```python
from build123d import *

# Parameters (mm, degrees)
RESSALTO_EXTRUS_O1_DEPTH = 70
RESSALTO_EXTRUS_O2_REACH = 92.865
CORTE_EXTRUS_O1_DEPTH    = 70


with BuildPart() as part:
    # Esboço1 → Ressalto-extrusão1 (new body)
    with BuildSketch(Plane.XY):
        Polygon((-46.166666667, -15.652777778), (33.833333333, 19.347222222), (33.833333333, -15.652777778), align=None)
    extrude(amount=RESSALTO_EXTRUS_O1_DEPTH)

    # Ressalto-extrusão2: up to this plane
    ressalto_extrus_o2_end = Plane(origin=(-46.166666667, -15.652777778, 70), z_dir=(0.4008188340197078, -0.9161573349021892, 0))
    # Esboço3 → Ressalto-extrusão2 (add, up to the surface)
    with BuildSketch(Plane.XZ.offset(15.652777778), mode=Mode.PRIVATE) as ressalto_extrus_o2_sk1:
        with BuildLine():
            Line((-10.666666667, 70), (-1.666666667, 70))
            Line((-1.666666667, 70), (-1.666666667, 75.846688069))
            ThreePointArc((-1.666666667, 75.846688069), (-6.166666667, 85.815315035), (-10.666666667, 75.846688069))
            Line((-10.666666667, 75.846688069), (-10.666666667, 70))
        make_face()
    ressalto_extrus_o2_tool1 = split(extrude(ressalto_extrus_o2_sk1.sketch, amount=-RESSALTO_EXTRUS_O2_REACH, mode=Mode.PRIVATE), bisect_by=ressalto_extrus_o2_end, keep=Keep.BOTH, mode=Mode.PRIVATE)
    add(ressalto_extrus_o2_tool1.solids().sort_by_distance((-6.166667, -15.652778, 77.842662))[0])

    # Esboço2 → Corte-extrusão1 (cut)
    with BuildSketch(Plane.XZ.offset(15.652777778)):
        with BuildLine():
            Line((-11.166666667, 0), (-1.166666667, 0))
            Line((-1.166666667, 0), (-1.166666667, 5.846688069))
            ThreePointArc((-1.166666667, 5.846688069), (-6.166666667, 16.5), (-11.166666667, 5.846688069))
            Line((-11.166666667, 5.846688069), (-11.166666667, 0))
        make_face()
    extrude(amount=-CORTE_EXTRUS_O1_DEPTH, mode=Mode.SUBTRACT)


solid = part.part
```
The listing builds one solid part. Answer for the finished solid, in the listing's coordinates (mm). A direction names the side the tool comes from. Give positions to 0.01 mm unless a question says otherwise; leave off trailing zeros. Loops run counter-clockwise (first coordinate to the right, second up) from the corner with the lowest first, then second, coordinate; pieces in that order, holes last. Notation, with made-up numbers: (41, -24.5) - (58, -24.5) arc R12 ccw to (58, -12.5) - close; hole circle Ø9 at (87.25, -5). An arc over 180 degrees is marked (long way). Return JSON: item names as keys, results as strings. Group by question number.
1. Straight lines are drawn through the part: line 1 (X direction, y = -14, z = 15); line 2 (Z direction, x = 7, y = 4); line 3 (X direction, y = -7.5, z = 16). For each, find the intervals that lie inside material, in ascending order. Write a range as [from, to].
2. Given pin 1 Ø1.8 at (y, z) = (-2.5, 2) entering from -X; pin 2 Ø6.5 at (y, z) = (-3, 74) entering from +X; pin 3 Ø10 at (x, z) = (-36.5, 43) entering from +Y, each flat-ended and moving along its own axis, determine where each tip first touches the part or whether it passes through.
3. Find section D-D (z = 44.5). Write down the section's boundary in (x, y), then the cut area to 3 significant figures.
4. Which of the six approach directions +Z, -Z, +X, -X, +Y, -Y give full straight-line access (tool end or side, diameter ignored) to faces 1 (the flat face through (-1.667, -6, 73)), 2 (the flat face through (-1.167, -6, 3)), 3 (the cylindrical face through (-3.073, -7.945, 84.956))?
5. Find section A-A (z = 10). Write down the section's boundary in (x, y).
6. Find section C-C (z = 74). Write down the section's boundary in (x, y), then the cut area to 4 significant figures.
7. Find section B-B (x = 18.5). Write down the section's boundary in (y, z).
8. Determine the mould class of faces 4 (the cylindrical face through (-5.961, -7.832, 16.497)), 5 (the flat face through (-10.667, -8, 73)), 6 (the flat face through (-21, -11, 0)), 7 (the flat face through (-11.167, -8, 3)) for opening direction Z: pulls with the +Z half, pulls with the -Z half, needs draft (parallel to the pull), parting line crosses it, or undercut.
Verdict:
{
 "1": {"line 1": "x = [-42.39, -10.32], [-2.01, 33.83]", "line 2": "z = [0, 70]", "line 3": "x = [-27.53, -8.67], [-3.67, 33.83]"},
 "2": {"pin 1": "stops at x = -18.16", "pin 2": "stops at x = -0.74", "pin 3": "stops at y = -9.24"},
 "3": {"outline": "(-46.17, -15.65) - (33.83, -15.65) - (33.83, 19.35) - close", "area": "1,400 mm^2"},
 "4": {"face 1": "+X, +Y, -Y", "face 2": "-Z, +Y, -Y", "face 3": "+Y, -Y"},
 "5": {"outline": "(-46.17, -15.65) - (-12.67, -15.65) - (-12.67, -1) - close; (0.33, -15.65) - (33.83, -15.65) - (33.83, 19.35) - (0.33, 4.69) - close"},
 "6": {"outline": "(-10.67, -15.65) - (-1.67, -15.65) - (-1.67, 3.82) - (-10.67, -0.12) - close", "area": "157.5 mm^2"},
 "7": {"outline": "(-15.65, 0) - (12.64, 0) - (12.64, 70) - (-15.65, 70) - close"},
 "8": {"face 4": "undercut", "face 5": "undercut", "face 6": "pulls with the -Z half", "face 7": "needs draft"}
}
